Build history of the part. All positions in model axes, mm. Face numbers are marked on the shaded views. A direction names the side the tool comes from. Give positions to 0.01 mm unless a question says otherwise; leave off trailing zeros. Order: outer loops, then holes, each group sorted by start corner. A loop starts at its lowest first (then second) coordinate and runs counter-clockwise, first axis right, second up. Notation, with made-up numbers: M 89,-10 L 97,-10 A5 cw 97,-2 Z; hole C -39.5,60.5 d2. An arc over 180 degrees is marked long. One line per item, written item: value.
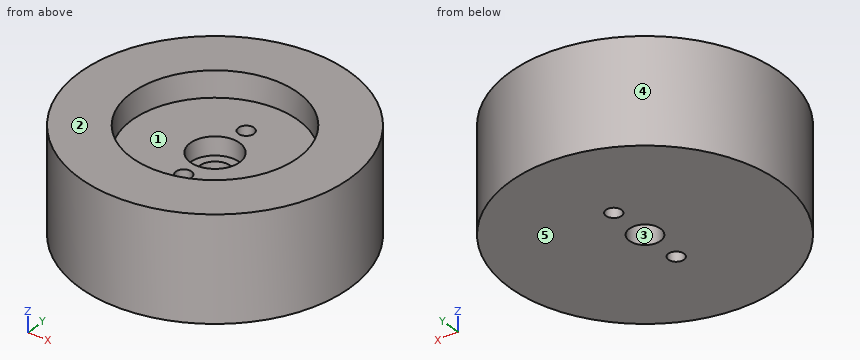
from build123d import *

# Parameters (mm, degrees)
ESQUISSE1_R             = 26
ESQUISSE1_R_2           = 3
BOSS_EXTRU_1_DEPTH      = 20
ESQUISSE2_R             = 16
ENL_V_MAT_EXTRU_1_DEPTH = 5
ESQUISSE3_R             = 4.75
ENL_V_MAT_EXTRU_2_DEPTH = 3.5
ESQUISSE4_R             = 1.5
ENL_V_MAT_EXTRU_3_DEPTH = 16


with BuildPart() as part:
    # Esquisse1 → Boss.-Extru.1 (new body)
    with BuildSketch(Plane.XY):
        Circle(ESQUISSE1_R)
        Circle(ESQUISSE1_R_2, mode=Mode.SUBTRACT)
    extrude(amount=BOSS_EXTRU_1_DEPTH)

    # Esquisse2 → Enlèv. mat.-Extru.1 (cut)
    with BuildSketch(Plane.XY.offset(20)):
        Circle(ESQUISSE2_R)
    extrude(amount=-ENL_V_MAT_EXTRU_1_DEPTH, mode=Mode.SUBTRACT)

    # Esquisse3 → Enlèv. mat.-Extru.2 (cut)
    with BuildSketch(Plane.XY.offset(15)):
        Circle(ESQUISSE3_R)
    extrude(amount=-ENL_V_MAT_EXTRU_2_DEPTH, mode=Mode.SUBTRACT)

    # Esquisse4 → Enlèv. mat.-Extru.3 (cut, through all)
    with BuildSketch(Plane.XY.offset(15)):
        with Locations((0, 8)):
            Circle(ESQUISSE4_R)
        with Locations((0, -8)):
            Circle(ESQUISSE4_R)
    extrude(amount=-ENL_V_MAT_EXTRU_3_DEPTH, mode=Mode.SUBTRACT)


solid = part.part
1) Saw through at B-B, the plane z = 18.5. Write the cut outline in (x, y).
Check values:
outline: C 0,0 d52; hole C 0,0 d32
2) Saw through at A-A, the plane y = 0. Write the cut outline in (x, z).
Check values:
outline: M -26,0 L -3,0 L -3,11.5 L -4.75,11.5 L -4.75,15 L -16,15 L -16,20 L -26,20 Z; M 3,0 L 26,0 L 26,20 L 16,20 L 16,15 L 4.75,15 L 4.75,11.5 L 3,11.5 Z
3) Saw through at C-C, the plane z = 6. Write the cut outline in (x, y).
Check values:
outline: C 0,0 d52; hole C 0,0 d6; hole C 0,-8 d3; hole C 0,8 d3
4) Drill centre lines: probe 1 along Y at (x, z) = (0, 4.5); probe 2 along Y at (x, z) = (0, 13.8); probe 3 along Y at (x, z) = (0, 16.25). Where is each one in solid material? Low to high. Write a range as from..to.
Check values:
probe 1: -26..-9.5, -6.5..-3, 3..6.5, 9.5..26
probe 2: -26..-9.5, -6.5..-4.75, 4.75..6.5, 9.5..26
probe 3: -26..-16, 16..26
5) Saw through at D-D, the plane x = -8.5. Write the cut outline in (y, z).
Check values:
outline: M -24.57,0 L 24.57,0 L 24.57,20 L 13.56,20 L 13.56,15 L -13.56,15 L -13.56,20 L -24.57,20 Z
6) Tool access for the marked faces 1 and 2: list every direction of +Z, -Z, +X, -X, +Y, -Y with a clear straight run to the whole face (end or side of a thin tool).
Check values:
face 1: +Z
face 2: +Z, +X, -X, +Y, -Y
7) Pin check, flat tips, straight feed: pin 1 (7 mm diameter, centred on x = 0, y = 0, fed in from +Z); pin 2 (1.5 mm diameter, centred on x = 18.5, z = 16, fed in from -Y); pin 3 (5 mm diameter, centred on x = 9.5, z = 16.5, fed in from +Y); pin 4 (2.5 mm diameter, centred on x = 0, y = 8, fed in from -Z). Stop position of each tip, or through.
Check values:
pin 1: z = 11.5
pin 2: y = -19
pin 3: y = 25.04
pin 4: through
8) Mould opens along X. For the marked faces 3, 4 and 5 say: released by +X, released by -X, zero draft, split by the parting line, or undercut.
Check values:
face 3: undercut
face 4: split by the parting line
face 5: zero draft
